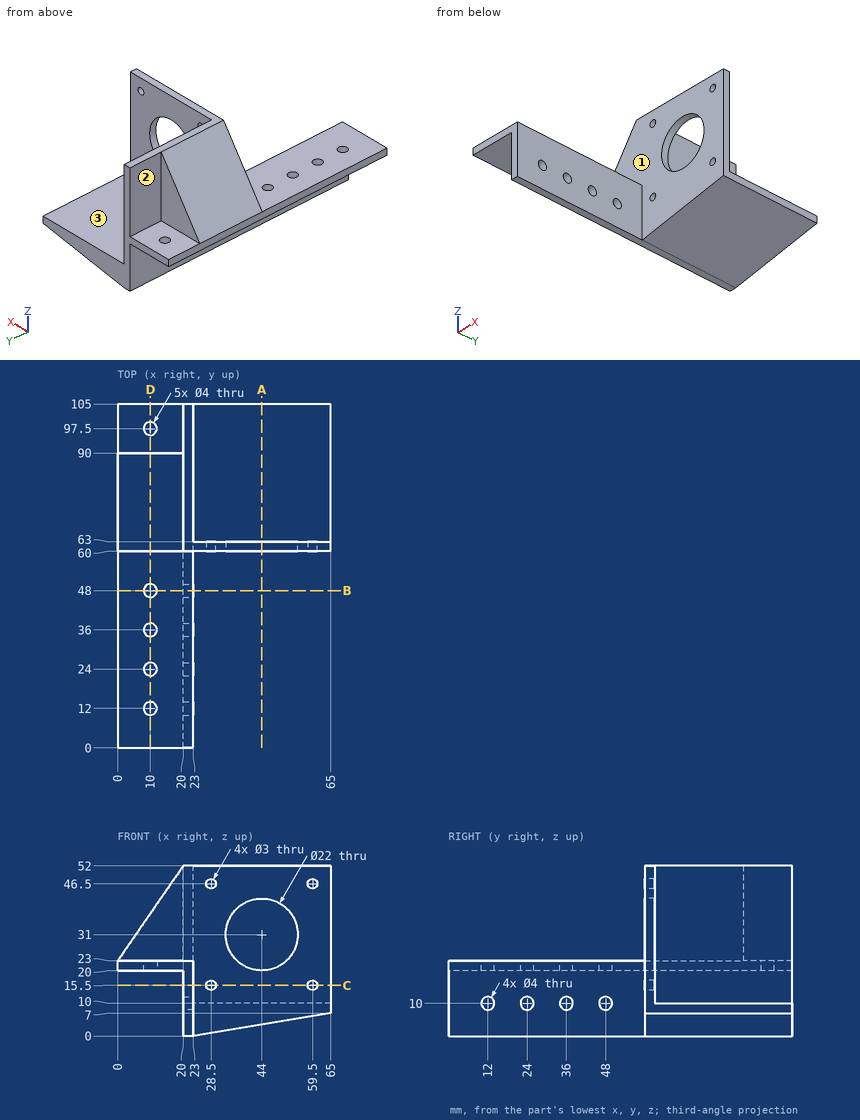
Print and shaded views of the part. All mm, measured from the part's lowest x, y and z. A direction names the side the tool comes from. Give positions to 0.01 mm unless a question says otherwise; leave off trailing zeros. Loops run counter-clockwise (first coordinate to the right, second up) from the corner with the lowest first, then second, coordinate; pieces in that order, holes last. Notation, with made-up numbers: (-23, 46) - (-8, 46) arc R13 ccw to (-8, 59) - close; hole circle Ø2 at (57, 45). An arc over 180 degrees is marked (long way). Use a Markdown table: item, result.
(1) Band-saw the part on D-D (x = 10). Give the cut face in (y, z).
Taken from the geometry:
| item | result |
|---|---|
| outline | (0, 20) - (10, 20) - (10, 23) - (0, 23) - close; (14, 20) - (22, 20) - (22, 23) - (14, 23) - close; (26, 20) - (34, 20) - (34, 23) - (26, 23) - close; (38, 20) - (46, 20) - (46, 23) - (38, 23) - close; (50, 20) - (95.5, 20) - (95.5, 23) - (90, 23) - (90, 37.5) - (60, 37.5) - (60, 23) - (50, 23) - close; (99.5, 20) - (105, 20) - (105, 23) - (99.5, 23) - close |
(2) Which spindle directions (+Z, -Z, +X, -X, +Y, -Y) get a long thin tool onto all of the face, cutting with end or side? Do the marked faces 1, 2 and 3. Say none if no direction does.
Taken from the geometry:
| item | result |
|---|---|
| face 1 | +Z, +X, -Y |
| face 2 | +Z, -X, +Y |
| face 3 | +Z, +X, +Y |
(3) Drop flat-ended pins along their axis: pin 1 Ø11.5 at (x, y) = (11.5, 32) entering from +Z; pin 2 Ø1 at (x, y) = (8, 39.5) entering from -Z; pin 3 Ø12 at (y, z) = (96.5, 41) entering from -X; pin 4 Ø12 at (x, y) = (27.5, 22) entering from -Z. Give the stop position or say it passes through.
Taken from the geometry:
| item | result |
|---|---|
| pin 1 | z = 23 |
| pin 2 | z = 20 |
| pin 3 | x = 20 |
| pin 4 | z = 0 |
(4) Wall check: line 1 along Y through (x, z) = (10, 22); line 2 along Z through (x, y) = (59, 61); line 3 along Z through (x, y) = (13, 15). Give the ranges that are in metal, low to high.
Taken from the geometry:
| item | result |
|---|---|
| line 1 | 0 to 10, 14 to 22, 26 to 34, 38 to 46, 50 to 95.5, 99.5 to 105 |
| line 2 | 6 to 14.09, 16.91 to 45.09, 47.91 to 52 |
| line 3 | 20 to 23 |
(5) Band-saw the part on A-A (x = 44). Give the cut face in (y, z).
Taken from the geometry:
| item | result |
|---|---|
| outline | (60, 3.5) - (105, 3.5) - (105, 10) - (63, 10) - (63, 20) - (60, 20) - close; (60, 42) - (63, 42) - (63, 52) - (60, 52) - close |
(6) Band-saw the part on C-C (z = 15.5). Give the cut face in (x, y), and give its area (3 significant figures).
Taken from the geometry:
| item | result |
|---|---|
| outline | (20, 0) - (23, 0) - (23, 60) - (27, 60) - (27, 63) - (23, 63) - (23, 105) - (20, 105) - close; (30, 60) - (58, 60) - (58, 63) - (30, 63) - close; (61, 60) - (65, 60) - (65, 63) - (61, 63) - close |
| area | 423 mm2 |
(7) Band-saw the part on B-B (y = 48). Give the cut face in (x, z).
Taken from the geometry:
| item | result |
|---|---|
| outline | (0, 20) - (8, 20) - (8, 23) - (0, 23) - close; (12, 20) - (20, 20) - (20, 12) - (23, 12) - (23, 23) - (12, 23) - close; (20, 0) - (23, 0) - (23, 8) - (20, 8) - close |
